```python
from build123d import *

# Parameters (mm, degrees)
BOSS_EXTRU_1_DEPTH           = 10
ENL_V_MAT_EXTRU_1_DEPTH      = 29.854594898
ENL_V_MAT_EXTRU_1_DEPTH_BACK = 29.854594898
ESQUISSE2_R                  = 2
ENL_V_START                  = 4
ESQUISSE3_R                  = 6
ENL_V_MAT_EXTRU_2_DEPTH      = 25.390139133
BOSS_EXTRU_2_REACH           = 35.257
ENL_V_START_2                = -20
ESQUISSE7_R                  = 1.2
ESQUISSE7_R_2                = 6
ENL_V_MAT_EXTRU_4_DEPTH      = 20
CONG_1_START                 = -10
CONG_1_DEPTH                 = 20
CONG_1_2_DEPTH               = 20
CONG_1_3_DEPTH               = 4.545644043
CONG_1_START_2               = 5.454355957
CONG_1_4_DEPTH               = 4.545644043
CONG_1_START_3               = -7
CONG_1_5_DEPTH               = 14
CONG_1_START_4               = 5.752776733
CONG_1_6_OUTLINE_R           = 6
CONG_1_6_DEPTH               = 28.247223267
CONG_1_START_5               = -1.5
CONG_1_7_DEPTH               = 8.118802154
BOSS_EXTRU_3_DEPTH           = 4
ENL_V_MAT_EXTRU_5_DEPTH      = 2
CONG_2_R                     = 1
CONG_3_R                     = 1
ENL_V_START_3                = -3
ENL_V_MAT_EXTRU_6_DEPTH      = 6
CONG_4_R                     = 8


with BuildPart() as part:
    # Esquisse1 → Boss.-Extru.1 (new, symmetric)
    with BuildSketch(Plane(origin=(0, 0, 0), x_dir=(1, 0, 0), z_dir=(0, 1, 0))):
        Polygon((2.35, 0), (9, 0), (9, -2), (1, -6.618802154), (1, -25), (-9, -25), (-9, 0), (-2.35, 0), (-2.35, 1.5), (2.35, 1.5), align=None)
    extrude(amount=BOSS_EXTRU_1_DEPTH, both=True)

    # Esquisse2 → Enlèv. mat.-Extru.1 (cut, two sides: drawn at the far end of the back side and taken through both)
    with BuildSketch(Plane(origin=(-1.372446517, 0, 0), x_dir=(1, 0, 0), z_dir=(0, 0, 1)).offset(-ENL_V_MAT_EXTRU_1_DEPTH_BACK)):
        with Locations((1.372446517, 0)):
            Circle(ESQUISSE2_R)
    extrude(amount=ENL_V_MAT_EXTRU_1_DEPTH + ENL_V_MAT_EXTRU_1_DEPTH_BACK, mode=Mode.SUBTRACT)

    # Esquisse3 → Enlèv. mat.-Extru.2 (cut, through all)
    with BuildSketch(Plane.XY.offset(ENL_V_START)):
        Circle(ESQUISSE3_R)
    extrude(amount=ENL_V_MAT_EXTRU_2_DEPTH, mode=Mode.SUBTRACT)

    # Boss.-Extru.2: up to this face of the body (flat: up to its plane)
    boss_extru_2_end = Plane(part.part.faces().sort_by_distance((-2.923443816, -10, 10.980550797))[0])
    # Esquisse6 → Boss.-Extru.2 (add, up to the picked face)
    with BuildSketch(Plane(origin=(0, 10, 0), x_dir=(1, 0, 0), z_dir=(0, 1, 0)), mode=Mode.PRIVATE) as boss_extru_2_sk1:
        Polygon((-9, -18.452994616), (5.803847577, -27), (15, -27), (15, -33), (-3.803847577, -33), (-9, -30), align=None)
    boss_extru_2_tool1 = split(extrude(boss_extru_2_sk1.sketch, amount=-BOSS_EXTRU_2_REACH, mode=Mode.PRIVATE), bisect_by=boss_extru_2_end, keep=Keep.BOTH, mode=Mode.PRIVATE)
    add(boss_extru_2_tool1.solids().sort_by(Axis((1.160347, 10, 28.066771), (0, -1, 0)))[0])

    # Esquisse7 → Enlèv. mat.-Extru.4 (cut)
    with BuildSketch(Plane.XY.offset(33).offset(ENL_V_START_2)):
        with Locations((10, 0)):
            Circle(ESQUISSE7_R)
        with Locations(Location((0, 0, 0), (0, 0, 230.656026391))):
            Circle(ESQUISSE7_R_2)
    extrude(amount=ENL_V_MAT_EXTRU_4_DEPTH, mode=Mode.SUBTRACT)

    # Congé1: read off the stored shape, not the designer's step
    # Congé1 outline → Congé1 (cut)
    with BuildSketch(Plane(origin=(0, 0, 0), x_dir=(1, 0, 0), z_dir=(0, 1, 0)).offset(CONG_1_START)):
        with BuildLine():
            Line((-9, -30), (-7.5, -30.866025404))
            ThreePointArc((-7.5, -30.866025404), (-8.598076211, -29.767949192), (-9, -28.267949192))
            Line((-9, -28.267949192), (-9, -30))
        make_face()
    extrude(amount=CONG_1_DEPTH, mode=Mode.SUBTRACT)

    # Cong_1 2 outline → Cong_1 2 (cut)
    with BuildSketch(Plane(origin=(0, 0, 0), x_dir=(1, 0, 0), z_dir=(0, 1, 0)).offset(CONG_1_START)):
        with BuildLine():
            Line((-3.803847577, -33), (-3, -33))
            ThreePointArc((-3, -33), (-3.776457135, -32.897777479), (-4.5, -32.598076211))
            Line((-4.5, -32.598076211), (-3.803847577, -33))
        make_face()
    extrude(amount=CONG_1_2_DEPTH, mode=Mode.SUBTRACT)

    # Cong_1 3 outline → Cong_1 3 (add)
    with BuildSketch(Plane(origin=(0, 0, 0), x_dir=(1, 0, 0), z_dir=(0, 1, 0)).offset(CONG_1_START)):
        with BuildLine():
            Line((5.803847577, -27), (6.607695155, -27))
            ThreePointArc((6.607695155, -27), (5.83123802, -26.897777479), (5.107695155, -26.598076211))
            Line((5.107695155, -26.598076211), (5.803847577, -27))
        make_face()
        with BuildLine():
            Line((1, -6.618802154), (1, -8.350852961))
            ThreePointArc((1, -8.350852961), (1.401923789, -6.850852961), (2.5, -5.75277675))
            Line((2.5, -5.75277675), (1, -6.618802154))
        make_face()
        with BuildLine():
            Line((1, -24.226497308), (2.5, -25.092522712))
            ThreePointArc((2.5, -25.092522712), (1.401923789, -23.994446501), (1, -22.494446501))
            Line((1, -22.494446501), (1, -24.226497308))
        make_face()
    extrude(amount=CONG_1_3_DEPTH)

    # Cong_1 4 outline → Cong_1 4 (add)
    with BuildSketch(Plane(origin=(0, 0, 0), x_dir=(1, 0, 0), z_dir=(0, 1, 0)).offset(CONG_1_START_2)):
        with BuildLine():
            Line((5.803847577, -27), (6.607695155, -27))
            ThreePointArc((6.607695155, -27), (5.83123802, -26.897777479), (5.107695155, -26.598076211))
            Line((5.107695155, -26.598076211), (5.803847577, -27))
        make_face()
        with BuildLine():
            Line((1, -6.618802154), (1, -8.350852961))
            ThreePointArc((1, -8.350852961), (1.401923789, -6.850852961), (2.5, -5.75277675))
            Line((2.5, -5.75277675), (1, -6.618802154))
        make_face()
        with BuildLine():
            Line((1, -24.226497308), (2.5, -25.092522712))
            ThreePointArc((2.5, -25.092522712), (1.401923789, -23.994446501), (1, -22.494446501))
            Line((1, -22.494446501), (1, -24.226497308))
        make_face()
    extrude(amount=CONG_1_4_DEPTH)

    # Cong_1 5 outline → Cong_1 5 (add)
    with BuildSketch(Plane(origin=(0, 0, 0), x_dir=(1, 0, 0), z_dir=(0, 1, 0)).offset(CONG_1_START_3)):
        with BuildLine():
            Line((5.803847577, -27), (6.607695155, -27))
            ThreePointArc((6.607695155, -27), (5.83123802, -26.897777479), (5.107695155, -26.598076211))
            Line((5.107695155, -26.598076211), (5.803847577, -27))
        make_face()
    extrude(amount=CONG_1_5_DEPTH)

    # Cong_1 6 outline → Cong_1 6 (cut)
    with BuildSketch(Plane.XY.offset(CONG_1_START_4)):
        with BuildLine():
            Line((-9, 10), (-9, 7))
            ThreePointArc((-9, 7), (-8.121320344, 9.121320344), (-6, 10))
            Line((-6, 10), (-9, 10))
        make_face()
        with BuildLine():
            ThreePointArc((-6, -10), (-8.121320344, -9.121320344), (-9, -7))
            Line((-9, -7), (-9, -10))
            Line((-9, -10), (-6, -10))
        make_face()
        with BuildLine():
            Line((15, -10), (15, -7))
            ThreePointArc((15, -7), (14.121320344, -9.121320344), (12, -10))
            Line((12, -10), (15, -10))
        make_face()
        Circle(CONG_1_6_OUTLINE_R)
    extrude(amount=CONG_1_6_DEPTH, mode=Mode.SUBTRACT)

    # Cong_1 7 outline → Cong_1 7 (cut)
    with BuildSketch(Plane.XY.offset(CONG_1_START_5)):
        with BuildLine():
            Line((-9, 10), (-9, 7))
            ThreePointArc((-9, 7), (-8.121320344, 9.121320344), (-6, 10))
            Line((-6, 10), (-9, 10))
        make_face()
        with BuildLine():
            ThreePointArc((-6, -10), (-8.121320344, -9.121320344), (-9, -7))
            Line((-9, -7), (-9, -10))
            Line((-9, -10), (-6, -10))
        make_face()
        with BuildLine():
            Line((9, 10), (6, 10))
            ThreePointArc((6, 10), (8.121320344, 9.121320344), (9, 7))
            Line((9, 7), (9, 10))
        make_face()
        with BuildLine():
            ThreePointArc((9, -7), (8.121320344, -9.121320344), (6, -10))
            Line((6, -10), (9, -10))
            Line((9, -10), (9, -7))
        make_face()
    extrude(amount=CONG_1_7_DEPTH, mode=Mode.SUBTRACT)

    # Esquisse8 → Boss.-Extru.3 (add)
    with BuildSketch(Plane.XZ.offset(10)):
        Polygon((-2.35, 0), (32.15767665, 0), (41, 33), (-2.35, 33), align=None)
    extrude(amount=-BOSS_EXTRU_3_DEPTH)

    # Esquisse9 → Enlèv. mat.-Extru.5 (cut)
    with BuildSketch(Plane.XZ.offset(10)):
        Polygon((-9, 1.5), (29.453771897, 1.5), (37.894171459, 33), (39.447085729, 33), (30.202838591, -1.5), (-9, -1.5), align=None)
    extrude(amount=-ENL_V_MAT_EXTRU_5_DEPTH, mode=Mode.SUBTRACT)

    # Congé2
    cong_2_edges = [part.edges().sort_by_distance(p)[0] for p in [
        (39.447085729, -9, 33),
        (29.453771897, -9, 1.5),
        (32.15767665, -8, 0),
        (36.578838325, -6, 16.5),
        (15, -6, 30),
        (20.578838325, -6, 0),
    ]]
    fillet(cong_2_edges, radius=CONG_2_R)

    # Congé3
    cong_3_edges = [part.edges().sort_by_distance(p)[0] for p in [
        (9, -6, 1.5),
        (9, -6.292893219, 0.292893219),
    ]]
    fillet(cong_3_edges, radius=CONG_3_R)

    # Esquisse10 → Enlèv. mat.-Extru.6 (cut)
    with BuildSketch(Plane.XY.offset(33).offset(ENL_V_START_3)):
        Polygon((12.75, 1.58771324), (10, 3.175426481), (7.25, 1.58771324), (7.25, -1.58771324), (10, -3.175426481), (12.75, -1.58771324), align=None)
    extrude(amount=-ENL_V_MAT_EXTRU_6_DEPTH, mode=Mode.SUBTRACT)

    # Congé4
    cong_4_edges = [part.edges().sort_by_distance(p)[0] for p in [
        (15, 10, 30),
    ]]
    fillet(cong_4_edges, radius=CONG_4_R)


solid = part.part
```
Input: part model. Units: mm. Frame: model coordinates. A direction names the side the tool comes from. Round coordinates to 2 decimals unless told otherwise and drop trailing zeros. Loops run counter-clockwise (first coordinate to the right, second up) from the corner with the lowest first, then second, coordinate; pieces in that order, holes last. Notation, with made-up numbers: (56.25, -30) -> (94.25, -30) arc R23 ccw to (94.25, -9) -> close; hole circle Ø5 at (5, 46.25). An arc over 180 degrees is marked (long way). One line per item, written item: value.
(1) Section A-A (y = 4.5). Return the cut outline in (x, z).
Geometry check:
outline: (-9, 0) -> (-2.35, 0) -> (-2.35, -1.5) -> (2.35, -1.5) -> (2.35, 0) -> (9, 0) -> (9, 2) -> (3.97, 4.9) -> (3.97, 4) -> (-3.97, 4) -> (-3.97, 32.84) arc R3 ccw to (-4.5, 32.6) -> (-7.5, 30.87) arc R3 ccw to (-9, 28.27) -> close; (3.97, 25.94) -> (5.11, 26.6) arc R3 cw to (6.61, 27) -> (14.6, 27) -> (14.6, 33) -> (3.97, 33) -> close
(2) Mould query, pull axis X, two halves, no side actions, for faces 4 (the face through (36.618, -8.521, 16.645)), 5 (the face through (7.25, 0, 29)), 6 (the face through (-6.312, 0.14, 31.552)). Classes: pulls with the +X half, pulls with the -X half, needs draft (parallel to the pull), parting line crosses it, or undercut.
Geometry check:
face 4: pulls with the +X half
face 5: undercut
face 6: pulls with the -X half
(3) Set-up query: faces 1 (the face through (-6, 1, 0)), 2 (the face through (6.01, 1.89, 26.94)), 3 (the face through (8, -1, 0)). Return all of +Z, -Z, +X, -X, +Y, -Y with unobstructed straight access to the full face (end or side cutting, diameter ignored); none if empty.
Geometry check:
face 1: -Z, -X, +Y, -Y
face 2: +X, +Y
face 3: -Z, +X, +Y, -Y
(4) Section B-B (x = 23). Return the cut outline in (y, z).
Geometry check:
outline: (-10, 1.5) -> (-8, 1.5) -> (-8, 0) -> (-7, 0) arc R1 ccw to (-6, 1) -> (-6, 33) -> (-10, 33) -> close
(5) Material intervals for line 1 (Y direction, x = 1, z = 24); line 2 (X direction, y = 0, z = 30.7); line 3 (Y direction, x = 0, z = 12), sorted ascending. Write a range as [from, to].
Geometry check:
line 1: [-10, -5.92], [5.92, 10]
line 2: [-7.76, -6], [6, 8.8], [11.2, 15]
line 3: [-10, -6], [6, 10]
(6) Pin query (flat end, axial travel): pin 1 (1.6 mm diameter, centred on x = 7.5, y = -9.5, fed in from -Z); pin 2 (1 mm diameter, centred on x = 31.5, z = 9.5, fed in from +Y); pin 3 (2 mm diameter, centred on y = 0.5, z = 1.5, fed in from +X). Return the tip coordinate at first contact, or that it passes through.
Geometry check:
pin 1: z = 1.5
pin 2: y = -6
pin 3: x = 9
(7) Section C-C (y = 8.25). Return the cut outline in (x, z), plus the area to 3 significant figures.
Geometry check:
outline: (-8.73, 0) -> (-2.35, 0) -> (-2.35, -1.5) -> (2.35, -1.5) -> (2.35, 0) -> (8.73, 0) -> (8.73, 2.16) -> (2.5, 5.75) arc R3 cw to (1, 8.35) -> (1, 22.49) arc R3 cw to (2.5, 25.09) -> (5.11, 26.6) arc R3 cw to (6.61, 27) -> (11.99, 27) -> (11.99, 33) -> (-3, 33) arc R3 ccw to (-4.5, 32.6) -> (-7.5, 30.87) arc R3 ccw to (-8.73, 29.52) -> close
area: 428 mm2
